Build history of the part. All positions in model axes, mm. Give positions to 0.01 mm unless a question says otherwise; leave off trailing zeros. Write each loop counter-clockwise with the first axis right and the second up, starting at its lowest first coordinate (ties: lowest second). Pieces come first, ordered by that corner, then holes. Notation, with made-up numbers: (20.25, 38) -> (26.25, 38) arc R19 ccw to (26.25, 52) -> close; hole circle Ø9 at (47, 72.25). An arc over 180 degrees is marked (long way). Write item = value, one per line. Start each with the question number.
Q1. Drop flat-ended pins along their axis: P1, Ø0.8, axis at x = -59.5, z = 0.5, coming from the -Y side; P2, Ø0.8, axis at y = 26, z = 1, coming from the -X side; P3, Ø0.8, axis at x = 6.5, z = 0.5, coming from the -Y side. Give the stop position or say it passes through.
Q2. Wall check: line 1 (Y direction, x = -39.5, z = 1.05); line 2 (X direction, y = 78.5, z = 1.05); line 3 (Y direction, x = -9, z = 0.9). Give the ranges that are in metal, low to high.
Q3. Saw through at A-A, the plane y = 24. List the corners of the cut face in (x, z), then the cut area to 3 significant figures.
Q4. Saw through at B-B, the plane x = 25. List the corners of the cut face in (y, z), then the cut area to 3 significant figures.
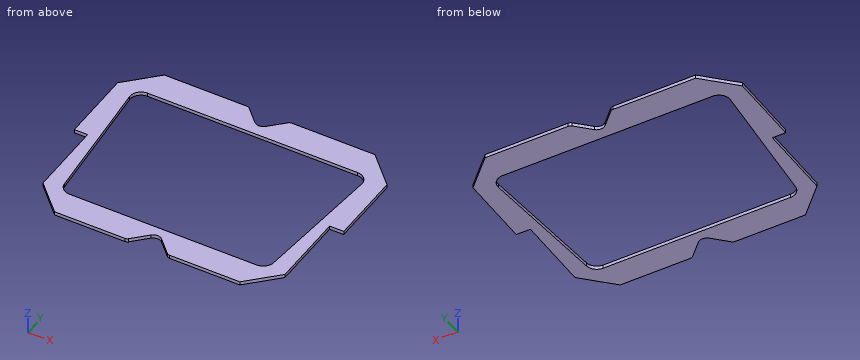
from build123d import *

# Parameters (mm, degrees)
EXTRUSION1_DEPTH = 1.6


with BuildPart() as part:
    # Esquisse1 → Extrusion1 (new body)
    with BuildSketch(Plane.XY):
        with BuildLine():
            Line((-48.023369217, 96.349184509), (-10.278174593, 96.349184509))
            ThreePointArc((-10.278174593, 96.349184509), (-9.512807728, 96.196943574), (-8.863961031, 95.763398071))
            Line((-8.863961031, 95.763398071), (-2.474873734, 89.374310774))
            ThreePointArc((-2.474873734, 89.374310774), (0, 88.349184509), (2.474873734, 89.374310774))
            Line((2.474873734, 89.374310774), (8.863961031, 95.763398071))
            ThreePointArc((8.863961031, 95.763398071), (9.512807728, 96.196943574), (10.278174593, 96.349184509))
            Line((10.278174593, 96.349184509), (48.369947474, 96.349184509))
            Line((48.369947474, 96.349184509), (61.879867656, 82.839264327))
            Line((61.879867656, 82.839264327), (61.879867656, 49.32839662))
            Line((61.879867656, 49.32839662), (55.4, 49.32839662))
            Line((55.4, 49.32839662), (55.4, 14.727514678))
            Line((55.4, 14.727514678), (42.421669831, 1.749184509))
            Line((42.421669831, 1.749184509), (10.278174593, 1.749184509))
            ThreePointArc((10.278174593, 1.749184509), (9.512807728, 1.901425444), (8.863961031, 2.334970946))
            Line((8.863961031, 2.334970946), (2.474873734, 8.724058243))
            ThreePointArc((2.474873734, 8.724058243), (0, 9.749184509), (-2.474873734, 8.724058243))
            Line((-2.474873734, 8.724058243), (-8.863961031, 2.334970946))
            ThreePointArc((-8.863961031, 2.334970946), (-9.512807728, 1.901425444), (-10.278174593, 1.749184509))
            Line((-10.278174593, 1.749184509), (-42.428554593, 1.749184509))
            Line((-42.428554593, 1.749184509), (-55.4, 14.720629916))
            Line((-55.4, 14.720629916), (-55.4, 49.32839662))
            Line((-55.4, 49.32839662), (-61.5, 49.32839662))
            Line((-61.5, 49.32839662), (-61.5, 82.872553726))
            Line((-61.5, 82.872553726), (-48.023369217, 96.349184509))
        make_face()
        with BuildLine():
            Line((-48.118530535, 83.349184509), (48.118530535, 83.349184509))
            ThreePointArc((48.118530535, 83.349184509), (51.805481915, 81.726519186), (53.099358035, 77.911740318))
            Line((53.099358035, 77.911740318), (47.891299628, 18.611740318))
            ThreePointArc((47.891299628, 18.611740318), (46.287806806, 15.362233129), (42.910472129, 14.049184509))
            Line((42.910472129, 14.049184509), (-42.910472129, 14.049184509))
            ThreePointArc((-42.910472129, 14.049184509), (-46.287806806, 15.362233129), (-47.891299628, 18.611740318))
            Line((-47.891299628, 18.611740318), (-53.099358035, 77.911740318))
            ThreePointArc((-53.099358035, 77.911740318), (-51.805481915, 81.726519186), (-48.118530535, 83.349184509))
        make_face(mode=Mode.SUBTRACT)
    extrude(amount=EXTRUSION1_DEPTH)


solid = part.part
Report:
q1.P1 = 49.33
q1.P2 = -55.4
q1.P3 = 4.3
q2.line_1 = 1.75 to 14.05, 83.35 to 96.35
q2.line_2 = -61.5 to -53.12, 53.12 to 61.88
q2.line_3 = 2.21 to 14.05, 83.35 to 95.89
q3.outline = (-55.4, 0) -> (-48.36, 0) -> (-48.36, 1.6) -> (-55.4, 1.6) -> close; (48.36, 0) -> (55.4, 0) -> (55.4, 1.6) -> (48.36, 1.6) -> close
q3.area = 22.5 mm2
q4.outline = (1.75, 0) -> (14.05, 0) -> (14.05, 1.6) -> (1.75, 1.6) -> close; (83.35, 0) -> (96.35, 0) -> (96.35, 1.6) -> (83.35, 1.6) -> close
q4.area = 40.5 mm2
